Autodesk Inventor part; units mm, degrees
ref_plane "YZ Plane" through (0, 0, 0) normal (1, 0, 0) x (0, 1, 0)
ref_plane "XZ Plane" through (0, 0, 0) normal (0, 1, 0) x (-1, 0, 0)
ref_plane "XY Plane" through (0, 0, 0) normal (0, 0, 1) x (1, 0, 0)
sketch "Sketch9" plane through (0, 0, 0) normal (0, 1, 0) x (-1, 0, 0)
  line L0 (15, 15) -> (-15, 15)
  line L1 (-15, 15) -> (-15, -15)
  line L2 (-15, -15) -> (15, -15)
  line L3 (15, -15) -> (15, 15)
  line L4 (15, 15) -> (-15, -15) construction
  line L5 (-15, 15) -> (15, -15) construction
  line L6 (-13, 13) -> (13, 13)
  line L7 (13, 13) -> (13, -13)
  line L8 (13, -13) -> (-13, -13)
  line L9 (-13, -13) -> (-13, 13)
  point P0 (0, 0)
  dimension "d172" = 30
  dimension "d173" = 30
  dimension "d174" = 2
extrude "Extrusion3" add sketch "Sketch9" against normal blind 320
sketch "Sketch10" plane through (0, 0, 0) normal (1, 0, 0) x (0, 1, 0)
  line L0 (0, 15) -> (0, -15) construction
  line L1 (0, 15) -> (-320, 15) construction
  line L2 (0, -15) -> (-320, -15) construction
  line L3 (-58.5, 8.5) -> (-41.5, 8.5)
  line L4 (-41.5, 8.5) -> (-41.5, -8.5)
  line L5 (-41.5, -8.5) -> (-58.5, -8.5)
  line L6 (-58.5, -8.5) -> (-58.5, 8.5)
  line L7 (-58.5, 8.5) -> (-41.5, -8.5) construction
  line L8 (-41.5, 8.5) -> (-58.5, -8.5) construction
  line L9 (0, 0) -> (30, 0)
  circle A0 centre (-50, 0) radius 8.5
  dimension "d177" = 17
  dimension "d178" = 17
  dimension "d181" = 30
  dimension "d182" = 80
extrude "Extrusion4" cut sketch "Sketch10" along normal through all contours A0
pattern_linear "Rectangular Pattern4" count 4 spacing 80 along (0, -1, 0) of "Extrusion4"
properties part number "PRS 1200-52-02 FDS 1000 way tube 2" material "Stainless Steel"
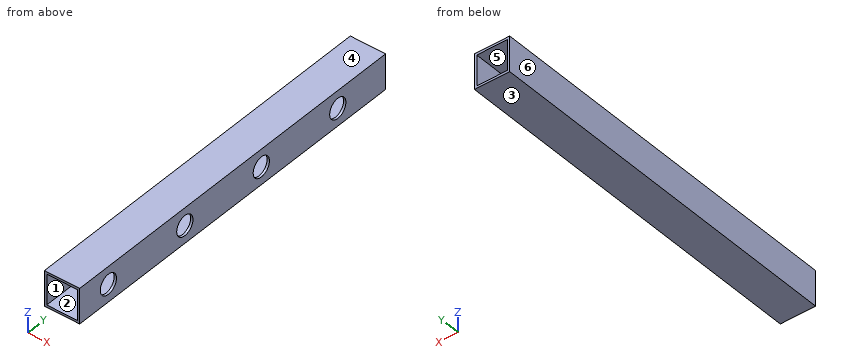
The listing builds one solid part. Answer for the finished solid, in the listing's coordinates (mm). Face numbers are marked on the shaded views. A direction names the side the tool comes from. Round coordinates to 2 decimals unless told otherwise and drop trailing zeros. Order: outer loops, then holes, each group sorted by start corner. A loop starts at its lowest first (then second) coordinate and runs counter-clockwise, first axis right, second up. Notation, with made-up numbers: (11, 16.5) -> (50, 16.5) arc R27 cw to (50, 37.5) -> close; hole circle Ø6 at (9, 38). An arc over 180 degrees is marked (long way). Put each result on its own line as item: value.
Q1. Which of the six approach directions +Z, -Z, +X, -X, +Y, -Y give full straight-line access (tool end or side, diameter ignored) to the marked faces 5 and 6?
Results list:
face 5: +Y, -Y
face 6: +Z, -Z, -X, +Y, -Y
Q2. Section C-C, the plane z = 5 is taken. Write down the section's boundary in (x, y), and give its area (3 significant figures).
Results list:
outline: (-15, -320) -> (-13, -320) -> (-13, 0) -> (-15, 0) -> close; (13, -320) -> (15, -320) -> (15, -296.87) -> (13, -296.87) -> close; (13, -283.13) -> (15, -283.13) -> (15, -216.87) -> (13, -216.87) -> close; (13, -203.13) -> (15, -203.13) -> (15, -136.87) -> (13, -136.87) -> close; (13, -123.13) -> (15, -123.13) -> (15, -56.87) -> (13, -56.87) -> close; (13, -43.13) -> (15, -43.13) -> (15, 0) -> (13, 0) -> close
area: 1,170 mm^2
Q3. Section A-A, the plane x = 8.75 is taken. Write down the section's boundary in (y, z), and give its area (3 significant figures).
Results list:
outline: (-320, -15) -> (0, -15) -> (0, -13) -> (-320, -13) -> close; (-320, 13) -> (0, 13) -> (0, 15) -> (-320, 15) -> close
area: 1,280 mm^2
Q4. Section B-B, the plane y = -28 is taken. Write down the section's boundary in (x, z), and give its area (3 significant figures).
Results list:
outline: (-15, -15) -> (15, -15) -> (15, 15) -> (-15, 15) -> close; hole (-13, -13) -> (13, -13) -> (13, 13) -> (-13, 13) -> close
area: 224 mm^2
Q5. Section D-D, the plane y = -210 is taken. Write down the section's boundary in (x, z).
Results list:
outline: (-15, -15) -> (15, -15) -> (15, -8.5) -> (13, -8.5) -> (13, -13) -> (-13, -13) -> (-13, 13) -> (13, 13) -> (13, 8.5) -> (15, 8.5) -> (15, 15) -> (-15, 15) -> close
Q6. Determine the mould class of the marked faces 1, 2, 3 and 4 for opening direction Z: pulls with the +Z half, pulls with the -Z half, needs draft (parallel to the pull), parting line crosses it, or undercut.
Results list:
face 1: undercut
face 2: undercut
face 3: pulls with the -Z half
face 4: pulls with the +Z half
Q7. Consider line 1 along Y through (x, z) = (14.05, 0); line 2 along X through (y, z) = (-162, 12.5). Determine where each line is inside the solid, lowest interval first.
Results list:
line 1: -320 to -298.5, -281.5 to -218.5, -201.5 to -138.5, -121.5 to -58.5, -41.5 to 0
line 2: -15 to -13, 13 to 15
